CAD build for the part. Positions are in the model's coordinates, mm. Round coordinates to 2 decimals unless told otherwise and drop trailing zeros. Write each loop counter-clockwise with the first axis right and the second up, starting at its lowest first coordinate (ties: lowest second). Pieces come first, ordered by that corner, then holes. Notation, with made-up numbers: (-5, -31) -> (17, -31) arc R28 ccw to (17, -10) -> close; hole circle Ø8 at (57.25, 45). An arc over 180 degrees is marked (long way). Put each result on its own line as item: value. Start each with the question number.
1. Saw through at C-C on y = 1.6. List the corners of the cut face in (x, z), and give its area (3 significant figures).
2. Saw through at A-A on x = 0. List the corners of the cut face in (y, z).
3. Saw through at B-B on z = 0. List the corners of the cut face in (x, y), and give its area (3 significant figures).
4. Drill centre lines: line 1 (X direction, y = 3.05, z = 0); line 2 (Z direction, x = 25.5, y = 1); line 3 (Z direction, x = 4, y = 0.4). Where is each one in solid material? Low to high. Write a range as from..to.
5. Flat gauge pin, fed straight in: P1, Ø2, axis at x = -27.5, y = 2.5, coming from the -Z side. Where does the tip first touch, or does it go through?
6. Saw through at D-D on z = -13. List the corners of the cut face in (x, y), and give its area (3 significant figures).
from build123d import *

# Parameters (mm, degrees)
SKETCH1_R           = 40
SKETCH1_R_2         = 5
BOSS_EXTRUDE1_DEPTH = 4
SKETCH2_W           = 5
SKETCH2_H           = 15
CUT_EXTRUDE1_DEPTH  = 4


with BuildPart() as part:
    # Sketch1 → Boss-Extrude1 (new body)
    with BuildSketch(Plane(origin=(0, 0, 0), x_dir=(1, 0, 0), z_dir=(0, 1, 0))):
        with Locations(Location((0, 0, 0), (0, 0, 270))):
            Circle(SKETCH1_R)
        with Locations(Location((0, 0, 0), (0, 0, 270))):
            Circle(SKETCH1_R_2, mode=Mode.SUBTRACT)
    extrude(amount=BOSS_EXTRUDE1_DEPTH)

    # Sketch2 → Cut-Extrude1 (cut)
    with BuildSketch(Plane(origin=(0, 4, 0), x_dir=(1, 0, 0), z_dir=(0, 1, 0))):
        with Locations((-27.5, 0)):
            Rectangle(SKETCH2_W, SKETCH2_H)
    cut_extrude1 = extrude(amount=-CUT_EXTRUDE1_DEPTH, mode=Mode.SUBTRACT)

    # Mirror1: Cut-Extrude1 across plane
    add(cut_extrude1.mirror(Plane(origin=(0, 0, 0), x_dir=(0, 0, 1), z_dir=(1, 0, 0))), mode=Mode.SUBTRACT)


solid = part.part
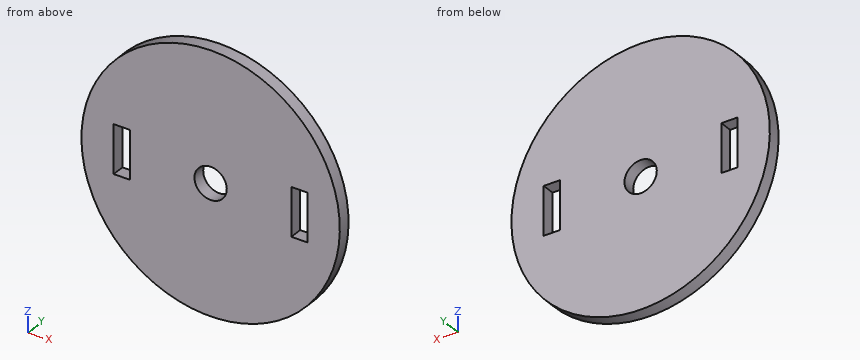
Return value:
1. outline: circle Ø80 at (0, 0); hole (-30, -7.5) -> (-25, -7.5) -> (-25, 7.5) -> (-30, 7.5) -> close; hole circle Ø10 at (0, 0); hole (25, -7.5) -> (30, -7.5) -> (30, 7.5) -> (25, 7.5) -> close
1. area: 4,800 mm^2
2. outline: (0, -40) -> (4, -40) -> (4, -5) -> (0, -5) -> close; (0, 5) -> (4, 5) -> (4, 40) -> (0, 40) -> close
3. outline: (-40, 0) -> (-30, 0) -> (-30, 4) -> (-40, 4) -> close; (-25, 0) -> (-5, 0) -> (-5, 4) -> (-25, 4) -> close; (5, 0) -> (25, 0) -> (25, 4) -> (5, 4) -> close; (30, 0) -> (40, 0) -> (40, 4) -> (30, 4) -> close
3. area: 240 mm^2
4. line 1: x = -40..-30, -25..-5, 5..25, 30..40
4. line 2: z = -30.82..-7.5, 7.5..30.82
4. line 3: z = -39.8..-3, 3..39.8
5. P1: stops at z = -29.96
6. outline: (-37.83, 0) -> (37.83, 0) -> (37.83, 4) -> (-37.83, 4) -> close
6. area: 303 mm^2
